```python
from build123d import *

# Parameters (mm, degrees)
SKETCH1_R           = 2
BOSS_EXTRUDE1_DEPTH = 3


with BuildPart() as part:
    # Sketch1 → Boss-Extrude1 (new body)
    with BuildSketch(Plane(origin=(0, 0, 0), x_dir=(1, 0, 0), z_dir=(0, 1, 0))):
        Polygon((0, 0), (-5, 0), (-5, 60), (5, 60), (5, 0), align=None)
        with Locations(Location((0, 20, 0), (0, 0, 270))):
            Circle(SKETCH1_R, mode=Mode.SUBTRACT)
        with Locations(Location((0, 5, 0), (0, 0, 270))):
            Circle(SKETCH1_R, mode=Mode.SUBTRACT)
        with Locations(Location((0, 50, 0), (0, 0, 270))):
            Circle(SKETCH1_R, mode=Mode.SUBTRACT)
    extrude(amount=BOSS_EXTRUDE1_DEPTH)


solid = part.part
```
The model under review builds one solid part; all positions refer to its coordinate system, in mm. Give positions to 0.01 mm unless a question says otherwise; leave off trailing zeros. Write each loop counter-clockwise with the first axis right and the second up, starting at its lowest first coordinate (ties: lowest second). Pieces come first, ordered by that corner, then holes. Notation, with made-up numbers: (74, 5.5) -> (95, 5.5) arc R18 cw to (95, 33.5) -> close; hole circle Ø9 at (59, 6.5). An arc over 180 degrees is marked (long way). Answer in a Markdown table with one row per item.
1) For L1, parallel to X at y = 2.3, z = -50; L2, parallel to Z at x = 0.75, y = 1.2; L3, parallel to Z at x = 1.75, y = 2.8, list the stretches that pass through material, from the lowest coordinate up. Write a range as [from, to].
Worked answers:
| item | result |
|---|---|
| L1 | [-5, -2], [2, 5] |
| L2 | [-60, -51.85], [-48.15, -21.85], [-18.15, -6.85], [-3.15, 0] |
| L3 | [-60, -50.97], [-49.03, -20.97], [-19.03, -5.97], [-4.03, 0] |
2) Add section A-A on z = -50. State the section outline as (x, y) points.
Worked answers:
| item | result |
|---|---|
| outline | (-5, 0) -> (-2, 0) -> (-2, 3) -> (-5, 3) -> close; (2, 0) -> (5, 0) -> (5, 3) -> (2, 3) -> close |
3) Add section B-B on x = 0. State the section outline as (y, z) points, plus the area to 3 significant figures.
Worked answers:
| item | result |
|---|---|
| outline | (0, -60) -> (3, -60) -> (3, -52) -> (0, -52) -> close; (0, -48) -> (3, -48) -> (3, -22) -> (0, -22) -> close; (0, -18) -> (3, -18) -> (3, -7) -> (0, -7) -> close; (0, -3) -> (3, -3) -> (3, 0) -> (0, 0) -> close |
| area | 144 mm² |
4) Mouldability with a two-part tool opening along Z and no side actions: class faces 1 (the flat face through (0, 1, 0)), 2 (the cylindrical face through (-1.2, 1.5, -21.6)), 3 (the flat face through (0, 1, -60)) as +Z half, -Z half, draft (parallel to the pull), parting line (faces both ways), or undercut.
Worked answers:
| item | result |
|---|---|
| face 1 | +Z half |
| face 2 | undercut |
| face 3 | -Z half |
5) Add section C-C on y = 0.5. State the section outline as (x, z) points.
Worked answers:
| item | result |
|---|---|
| outline | (-5, -60) -> (5, -60) -> (5, 0) -> (-5, 0) -> close; hole circle Ø4 at (0, -50); hole circle Ø4 at (0, -20); hole circle Ø4 at (0, -5) |
